```python
from build123d import *

# Parameters (mm, degrees)
F0_R     = 9.5
F1_DEPTH = 150
F2_DEPTH = 20
F3_DEPTH = 20
F4_DEPTH = 300
F5_DEPTH = 300


with BuildPart() as f1:
    # F0 (on Top) → F1 (new body)
    with BuildSketch(Plane.XY):
        with BuildLine():
            ThreePointArc((-74.9990347614, 0.3805060562), (-74.99975869, 0.1902536402), (-75, 0))
            ThreePointArc((-75, 0), (0, -75), (75, 0))
            ThreePointArc((75, 0), (0.1902536402, 74.99975869), (-74.9990347614, 0.3805060562))
        make_face()
        with BuildLine():
            ThreePointArc((-73.2942603105, 0), (-64.7942603105, 8.5738779646), (-56.2942603105, 0))
            ThreePointArc((-56.2942603105, 0), (-64.7942603105, -8.5), (-73.2942603105, 0))
        make_face(mode=Mode.SUBTRACT)
        with BuildLine():
            ThreePointArc((-55, 0), (-54.9998230393, 0.1395193362), (-54.9992921584, 0.2790377745))
            ThreePointArc((-54.9992921584, 0.2790377745), (0.1395193362, 54.9998230393), (55, 0))
            ThreePointArc((55, 0), (0, -55), (-55, 0))
        make_face(mode=Mode.SUBTRACT)
        with Locations((65.0509051438, 0)):
            Circle(F0_R, mode=Mode.SUBTRACT)
    extrude(amount=F1_DEPTH)

    # F0 (on Top) → F2 (join)
    with BuildSketch(Plane.XY):
        with BuildLine():
            ThreePointArc((-74.9990347614, 0.3805060562), (-74.99975869, 0.1902536402), (-75, 0))
            ThreePointArc((-75, 0), (0, -75), (75, 0))
            ThreePointArc((75, 0), (0.1902536402, 74.99975869), (-74.9990347614, 0.3805060562))
        make_face()
        with BuildLine():
            ThreePointArc((-73.2942603105, 0), (-64.7942603105, 8.5738779646), (-56.2942603105, 0))
            ThreePointArc((-56.2942603105, 0), (-64.7942603105, -8.5), (-73.2942603105, 0))
        make_face(mode=Mode.SUBTRACT)
        with BuildLine():
            ThreePointArc((-55, 0), (-54.9998230393, 0.1395193362), (-54.9992921584, 0.2790377745))
            ThreePointArc((-54.9992921584, 0.2790377745), (0.1395193362, 54.9998230393), (55, 0))
            ThreePointArc((55, 0), (0, -55), (-55, 0))
        make_face(mode=Mode.SUBTRACT)
        with Locations((65.0509051438, 0)):
            Circle(F0_R, mode=Mode.SUBTRACT)
        with BuildLine():
            ThreePointArc((-55, 0), (-54.998672885, 0.1395164185), (-54.9992921584, 0.2790377745))
            ThreePointArc((-54.9992921584, 0.2790377745), (-54.9998230393, 0.1395193362), (-55, 0))
        make_face()
        with BuildLine():
            ThreePointArc((55, 0), (0.1395193362, 54.9998230393), (-54.9992921584, 0.2790377745))
            ThreePointArc((-54.9992921584, 0.2790377745), (-54.998672885, 0.1395164185), (-55, 0))
            ThreePointArc((-55, 0), (0, -55), (55, 0))
        make_face()
    extrude(amount=F2_DEPTH)

    # F0 (on Top) → F3 (join)
    with BuildSketch(Plane.XY):
        with BuildLine():
            ThreePointArc((-73.2942603105, 0), (-64.7942603105, -8.5), (-56.2942603105, 0))
            ThreePointArc((-56.2942603105, 0), (-64.7942603105, 8.5), (-73.2942603105, 0))
        make_face()
        with Locations((65.0509051438, 0)):
            Circle(F0_R)
    extrude(amount=F3_DEPTH)

    # F4 (add): a face of the model
    f4_faces = [f1.faces().sort_by_distance(p)[0] for p in [
        (-64.7942603105, 0, 20),
    ]]
    extrude(f4_faces, amount=F4_DEPTH)

    # F5 (add): a face of the model
    f5_faces = [f1.faces().sort_by_distance(p)[0] for p in [
        (65.0509051438, 0, 20),
    ]]
    extrude(f5_faces, amount=F5_DEPTH)


solid = f1.part
```
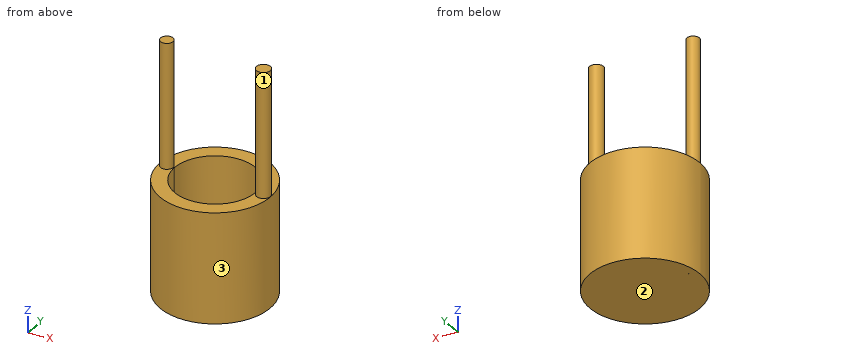
The model under review builds one solid part; all positions refer to its coordinate system, in mm. Face numbers are marked on the shaded views. Coordinates: 2 decimals unless noted, no trailing zeros. Write each loop counter-clockwise with the first axis right and the second up, starting at its lowest first coordinate (ties: lowest second). Pieces come first, ordered by that corner, then holes. Notation, with made-up numbers: (-32, 2.5) - (-19, 2.5) arc R29 ccw to (-19, 31.5) - close; hole circle Ø3 at (52, -11). An arc over 180 degrees is marked (long way). Answer in a Markdown table with one row per item. Add a question column.
Q1. Clearance check with flat-ended pins moving along their axes: pin 1 (5 mm diameter, centred on x = -10.5, y = -7, fed in from +Z); pin 2 (5 mm diameter, centred on x = 5.5, z = 36, fed in from +Y); pin 3 (5 mm diameter, centred on y = -43.5, z = 119.5, fed in from -X). State where each tip first meets the part, or that it passes through.
Q2. Consider section C-C on y = 47. Give the boundary of the cut face in (x, z), then the cut area to 3 significant figures.
Q3. Consider section D-D on y = -61. Give the boundary of the cut face in (x, z), then the cut area to 3 significant figures.
Q4. Consider section B-B on z = 191.5. Give the boundary of the cut face in (x, y), then the cut area to 3 significant figures.
Q5. To check wall thickness, follow line 1 along Y through (x, z) = (0, 99); line 2 along Z through (x, y) = (-19, -25.5); line 3 along Z through (x, y) = (-22.5, 53.5). State the ranges of each line that lie inside material, in increasing order. Write a range as from..to.
Q6. Draft analysis for pull direction X (two halves, no side actions). For the marked faces 1, 2 and 3, state which applies: +X half, -X half, draft (parallel to the pull), parting line (faces both ways), or undercut.
Q7. Consider section A-A on x = 0. Give the boundary of the cut face in (y, z), then the cut area to 3 significant figures.
Answers below:
| question | item | result |
|---|---|---|
| 1 | pin 1 | z = 20 |
| 1 | pin 2 | y = 74.94 |
| 1 | pin 3 | x = -62.8 |
| 2 | outline | (-58.45, 0) - (58.45, 0) - (58.45, 150) - (28.57, 150) - (28.57, 20) - (-28.57, 20) - (-28.57, 150) - (-58.45, 150) - close |
| 2 | area | 10,100 mm² |
| 3 | outline | (-43.63, 0) - (43.63, 0) - (43.63, 150) - (-43.63, 150) - close |
| 3 | area | 13,100 mm² |
| 4 | outline | circle Ø17 at (-64.79, 0); circle Ø19 at (65.05, 0) |
| 4 | area | 511 mm² |
| 5 | line 1 | -75..-55, 55..75 |
| 5 | line 2 | 0..20 |
| 5 | line 3 | 0..150 |
| 6 | face 1 | undercut |
| 6 | face 2 | draft |
| 6 | face 3 | parting line |
| 7 | outline | (-75, 0) - (75, 0) - (75, 150) - (55, 150) - (55, 20) - (-55, 20) - (-55, 150) - (-75, 150) - close |
| 7 | area | 8,200 mm² |
